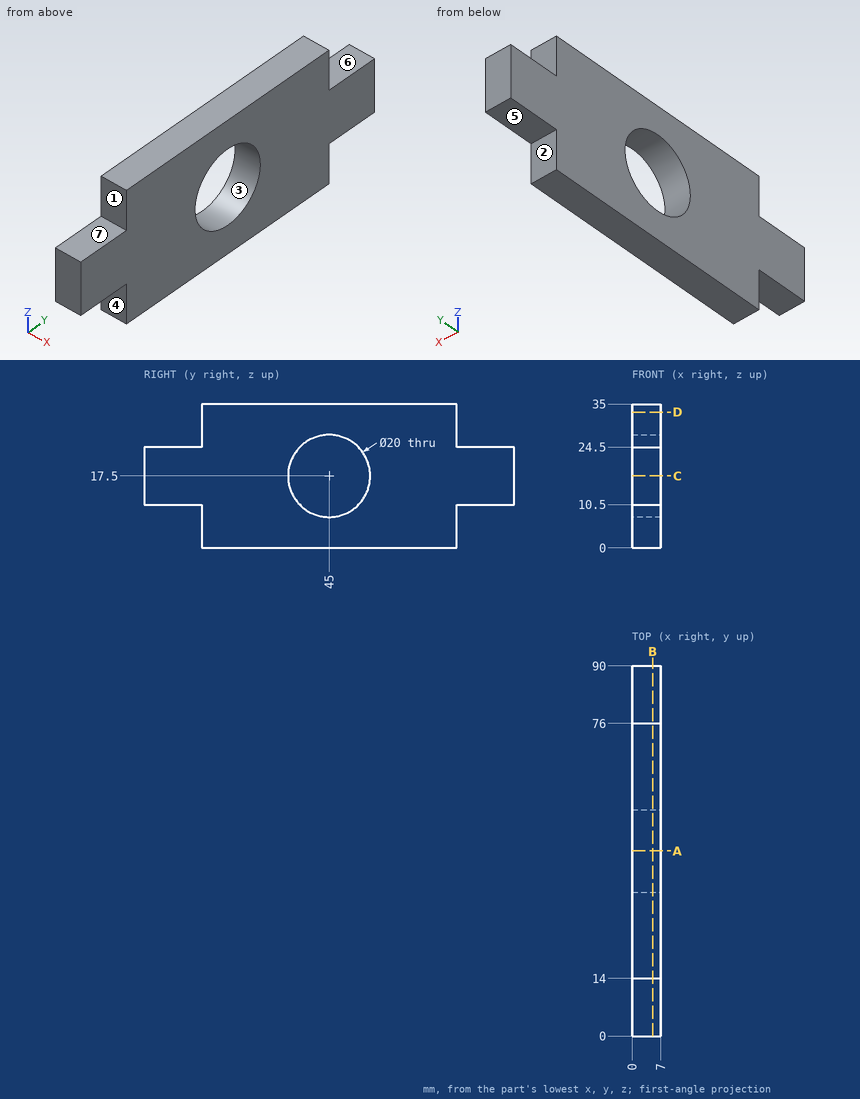
Check sheet for the drawn part. Datum: minimum x, y, z corner. Units: mm. A direction names the side the tool comes from. Coordinates: 2 decimals unless noted, no trailing zeros. Order: outer loops, then holes, each group sorted by start corner. A loop starts at its lowest first (then second) coordinate and runs counter-clockwise, first axis right, second up. Notation, with made-up numbers: (22.25, -4) -> (41.25, -4) arc R35 cw to (41.25, 34) -> close; hole circle Ø5 at (15.5, 24.5). An arc over 180 degrees is marked (long way). Write each question's results on one line, items separated by ' | '. Start each with the question number.
1) Depth check by flat-ended pin: pin 1 (4 mm diameter, centred on x = 1.5, z = 30.5, fed in from -Y); pin 2 (3.5 mm diameter, centred on x = 4, z = 3.5, fed in from +Y); pin 3 (12 mm diameter, centred on y = 45, z = 17.5, fed in from +X); pin 4 (4 mm diameter, centred on x = 3.5, y = 10.5, fed in from +Z). Enter the tip coordinate at first touch or a pass-through.
2) Section check C-C (z = 17.5). Enter the section's corners in (x, y), and give its area (3 significant figures).
3) Section check A-A (y = 45). Enter the section's corners in (x, z).
4) Section check D-D (z = 33). Enter the section's corners in (x, y), and give its area (3 significant figures).
5) Material ranges on line 1 along Y through (x, z) = (3.25, 17.5); line 2 along Y through (x, z) = (3, 5.5); line 3 along Z through (x, y) = (3.5, 50), recorded low to high.
6) Set-up check for the marked faces 4, 5, 6 and 7: record each of +Z, -Z, +X, -X, +Y, -Y from which the full face is reachable in a straight line by a thin tool's end or side.
7) Draft check along Y on the marked faces 1, 2 and 3. Enter one of: pulls with the +Y half, pulls with the -Y half, needs draft (parallel to the pull), parting line crosses it, or undercut.
8) Section check B-B (x = 5). Enter the section's corners in (y, z), and give its area (3 significant figures).
Checked values:
1) pin 1: y = 14 | pin 2: y = 76 | pin 3: through | pin 4: z = 24.5
2) outline: (0, 0) -> (7, 0) -> (7, 35) -> (0, 35) -> close; (0, 55) -> (7, 55) -> (7, 90) -> (0, 90) -> close | area: 490 mm²
3) outline: (0, 0) -> (7, 0) -> (7, 7.5) -> (0, 7.5) -> close; (0, 27.5) -> (7, 27.5) -> (7, 35) -> (0, 35) -> close
4) outline: (0, 14) -> (7, 14) -> (7, 76) -> (0, 76) -> close | area: 434 mm²
5) line 1: 0 to 35, 55 to 90 | line 2: 14 to 76 | line 3: 0 to 8.84, 26.16 to 35
6) face 4: -Z, +X, -X, -Y | face 5: -Z, +X, -X, +Y | face 6: +Z, +X, -X, +Y | face 7: +Z, +X, -X, -Y
7) face 1: pulls with the -Y half | face 2: pulls with the +Y half | face 3: undercut
8) outline: (0, 10.5) -> (14, 10.5) -> (14, 0) -> (76, 0) -> (76, 10.5) -> (90, 10.5) -> (90, 24.5) -> (76, 24.5) -> (76, 35) -> (14, 35) -> (14, 24.5) -> (0, 24.5) -> close; hole circle Ø20 at (45, 17.5) | area: 2,250 mm²
